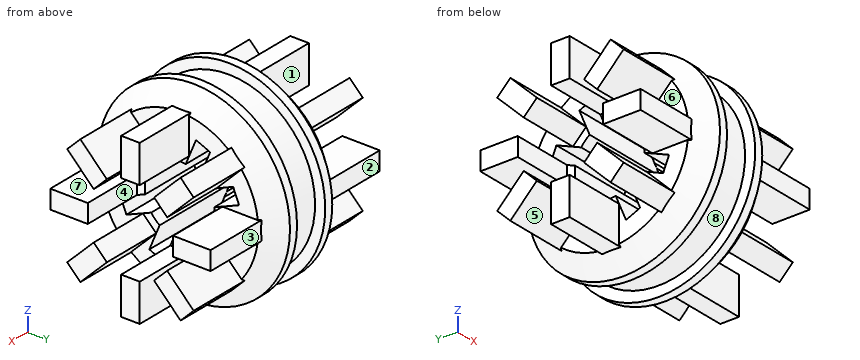
from build123d import *

# Parameters (mm, degrees)
SKETCH1_W               = 1.062231574
SKETCH1_H               = 2.14234413
SKETCH1_W_2             = 2.14234413
SKETCH1_H_2             = 1.062231574
BOSS_EXTRUDE3_DEPTH     = 6
CUT_EXTRUDE1_DEPTH      = 10.823441352
CUT_EXTRUDE1_DEPTH_BACK = 10.823441352


with BuildPart() as part:
    # Sketch3 → Revolve1 (revolve)
    with BuildSketch(Plane(origin=(0, 0, 0), x_dir=(1, 0, 0), z_dir=(0, 1, 0)), mode=Mode.PRIVATE) as revolve1_sk:
        Polygon((1, 5.5), (1.5, 5.5), (2.5, 4.5), (2.5, 2), (-2.5, 2), (-2.5, 4.5), (-1.5, 5.5), (-1, 5.5), (-1, 4.919351403), (1, 4.919351403), align=None)
    revolve(revolve1_sk.sketch.rotate(Axis((0, 0, 0), (1, 0, 0)), 180), axis=Axis((0, 0, 0), (1, 0, 0)))

    # Sketch1 → Boss-Extrude3 (add, symmetric)
    with BuildSketch(Plane(origin=(0, 0, 0), x_dir=(0, 0, -1), z_dir=(1, 0, 0))):
        Polygon((-3.617835313, -2.866724163), (-2.102969252, -1.351858102), (-1.351858102, -2.102969252), (-2.866724163, -3.617835313), align=None)
        with Locations((0, -3.514103914)):
            Rectangle(SKETCH1_W, SKETCH1_H)
        with Locations((-3.514103914, 0)):
            Rectangle(SKETCH1_W_2, SKETCH1_H_2)
        Polygon((-2.866724163, 3.617835313), (-1.351858102, 2.102969252), (-2.102969252, 1.351858102), (-3.617835313, 2.866724163), align=None)
        with Locations((0, 3.514103914)):
            Rectangle(SKETCH1_W, SKETCH1_H)
        Polygon((3.617835313, 2.866724163), (2.102969252, 1.351858102), (1.351858102, 2.102969252), (2.866724163, 3.617835313), align=None)
        with Locations((3.514103914, 0)):
            Rectangle(SKETCH1_W_2, SKETCH1_H_2)
        Polygon((2.866724163, -3.617835313), (1.351858102, -2.102969252), (2.102969252, -1.351858102), (3.617835313, -2.866724163), align=None)
    extrude(amount=BOSS_EXTRUDE3_DEPTH, both=True)

    # Sketch4 → Cut-Extrude1 (cut, two sides: drawn at the far end of the back side and taken through both)
    with BuildSketch(Plane(origin=(0, 0, 0), x_dir=(0, 0, -1), z_dir=(1, 0, 0)).offset(-CUT_EXTRUDE1_DEPTH_BACK)):
        Polygon((1.741274388, 3.054032834), (1.128980896, 1.575825582), (0.315966908, 1.912587003), (0.928260399, 3.390794255), align=None)
        Polygon((3.390794255, 0.928260399), (1.912587003, 0.315966908), (1.575825582, 1.128980896), (3.054032834, 1.741274388), align=None)
        Polygon((3.054032834, -1.741274388), (1.575825582, -1.128980896), (1.912587003, -0.315966908), (3.390794255, -0.928260399), align=None)
        Polygon((0.928260399, -3.390794255), (0.315966908, -1.912587003), (1.128980896, -1.575825582), (1.741274388, -3.054032834), align=None)
        Polygon((-1.741274388, -3.054032834), (-1.128980896, -1.575825582), (-0.315966908, -1.912587003), (-0.928260399, -3.390794255), align=None)
        Polygon((-3.390794255, -0.928260399), (-1.912587003, -0.315966908), (-1.575825582, -1.128980896), (-3.054032834, -1.741274388), align=None)
        Polygon((-3.054032834, 1.741274388), (-1.575825582, 1.128980896), (-1.912587003, 0.315966908), (-3.390794255, 0.928260399), align=None)
        Polygon((-0.928260399, 3.390794255), (-0.315966908, 1.912587003), (-1.128980896, 1.575825582), (-1.741274388, 3.054032834), align=None)
    extrude(amount=CUT_EXTRUDE1_DEPTH + CUT_EXTRUDE1_DEPTH_BACK, mode=Mode.SUBTRACT)


solid = part.part
Verification items for the finished model (mm, model axes). Face numbers are marked on the shaded views. A direction names the side the tool comes from. Give positions to 0.01 mm unless a question says otherwise; leave off trailing zeros.
1) Set-up check for the marked faces 1, 2, 3, 4 and 5: record each of +Z, -Z, +X, -X, +Y, -Y from which the full face is reachable in a straight line by a thin tool's end or side.
2) Draft check along X on the marked faces 6, 7 and 8. Enter one of: pulls with the +X half, pulls with the -X half, needs draft (parallel to the pull), parting line crosses it, or undercut.
3) Thickness scan on line 1 along Y through (x, z) = (-4.5, -0.5); line 2 along Z through (x, y) = (-5.5, -3); line 3 along Z through (x, y) = (-4.75, 2.75). Record the ranges inside material, lowest first.
4) Sectioned sample at A-A, the plane x = 4.5. Count the separate pieces of the cut face and the enclosed holes in it, then the cut area to 3 significant figures.
5) Depth check by flat-ended pin: pin 1 Ø1 at (y, z) = (-2.5, -4.5) entering from -X; pin 2 Ø0.5 at (x, y) = (4.5, 0) entering from +Z; pin 3 Ø1.2 at (x, z) = (4.5, 0) entering from -Y. Enter the tip coordinate at first touch or a pass-through.
Answers:
1. face 1: +Z, -Z, -X
1. face 2: +Z, -Z, -X, +Y
1. face 3: +Z, -Z, +X, +Y
1. face 4: +X
1. face 5: -Z, -X
2. face 6: pulls with the -X half
2. face 7: needs draft
2. face 8: undercut
3. line 1: y = -4.59 to -2.44, 2.44 to 4.59
3. line 2: z = -3.48 to -2.25, -0.53 to 0.53, 2.25 to 3.48
3. line 3: z = -3.5 to -2, -0.53 to 0.53, 2 to 3.5
4. separate pieces: 8
4. enclosed holes: 0
4. area: 18.2 mm2
5. pin 1: stops at x = -2.35
5. pin 2: stops at z = 4.59
5. pin 3: stops at y = -4.59
